```python
from build123d import *

# Parameters (mm, degrees)
SKETCH1_W           = 7.62
SKETCH1_H           = 7.62
BOSS_EXTRUDE1_DEPTH = 8.255
SKETCH3_R           = 1.5875
BOSS_EXTRUDE2_DEPTH = 6.35
SKETCH4_R           = 1.5875
BOSS_EXTRUDE3_DEPTH = 6.35


with BuildPart() as part:
    # Sketch1 → Boss-Extrude1 (new, symmetric)
    with BuildSketch(Plane.XY):
        Rectangle(SKETCH1_W, SKETCH1_H)
    extrude(amount=BOSS_EXTRUDE1_DEPTH, both=True)

    # Sketch2 → Cut-Revolve2 (revolve, cut)
    with BuildSketch(Plane(origin=(0, 0, 0), x_dir=(-1, 0, 0), z_dir=(0, -1, 0)), mode=Mode.PRIVATE) as cut_revolve2_sk:
        Polygon((-3.683, 8.255), (-12.573, 8.255), (-12.573, -8.255), (-3.683, -8.255), (-11.303, -3.855590949), (-11.303, 3.855590949), align=None)
    revolve(cut_revolve2_sk.sketch.rotate(Axis((0, 0, -8.255), (0, 0, 1)), 180), axis=Axis((0, 0, -8.255), (0, 0, 1)), mode=Mode.SUBTRACT)

    # Sketch3 → Boss-Extrude2 (add, symmetric)
    with BuildSketch(Plane.XZ):
        with Locations(Location((0, 0, 0), (0, 0, 90))):
            Circle(SKETCH3_R)
    extrude(amount=BOSS_EXTRUDE2_DEPTH, both=True)

    # Sketch4 → Boss-Extrude3 (add, symmetric)
    with BuildSketch(Plane.ZY):
        with Locations(Location((0, 0, 0), (0, 0, 180))):
            Circle(SKETCH4_R)
    extrude(amount=BOSS_EXTRUDE3_DEPTH, both=True)


solid = part.part
```
Can you work these out from the model? Positions are in its coordinate system, mm. A direction names the side the tool comes from. Coordinates: 2 decimals unless noted, no trailing zeros. Loops run counter-clockwise (first coordinate to the right, second up) from the corner with the lowest first, then second, coordinate; pieces in that order, holes last.
1) I need wall thicknesses on probe 1 along Y at (x, z) = (2.75, -0.25); probe 2 along X at (y, z) = (4.25, 1.25). Which ranges of each line are inside material? Lowest first, please.
2) Which directions (+Z, -Z, +X, -X, +Y, -Y) give clear straight access to the entire face, cutting with the end or side of a thin tool? Please do faces 1 (the cylindrical face through (5.06, 1.41, -0.73)), 2 (the flat face through (0, 6.35, 0)), 3 (the cylindrical face through (-5.1, 1.41, -0.73)), 4 (the cylindrical face through (0.966, -5.098, -1.26)), 5 (the cylindrical face through (0.966, 5.062, -1.26)).
3) Imagine slicing it at D-D on x = -5. List the corners of the cut face in (y, z) for me (1 decimal), plus the area to 3 significant figures.
4) Imagine slicing it at C-C on z = 0. List the corners of the cut face in (x, y) for me, plus the area to 3 significant figures.
5) For pin 1 (1 mm diameter, centred on x = 4.5, y = 0, fed in from -Z); pin 2 (4 mm diameter, centred on x = 4.5, y = -4, fed in from +Z); pin 3 (1.5 mm diameter, centred on y = 2, z = 2.5, fed in from -X), each with a flat end and sliding along its axis, tell me the tip position at first contact or that it passes through.
Completed:
1. probe 1: y = -3.81 to 3.81
1. probe 2: x = -0.98 to 0.98
2. face 1: +X
2. face 2: +Z, -Z, +X, -X, +Y
2. face 3: -X
2. face 4: -Y
2. face 5: +Y
3. outline: circle Ø3.2 at (0, 0)
3. area: 7.92 mm2
4. outline: (-6.35, -1.59) - (-3.81, -1.59) - (-3.81, -3.81) - (-1.59, -3.81) - (-1.59, -6.35) - (1.59, -6.35) - (1.59, -3.81) - (3.81, -3.81) - (3.81, -1.59) - (6.35, -1.59) - (6.35, 1.59) - (3.81, 1.59) - (3.81, 3.81) - (1.59, 3.81) - (1.59, 6.35) - (-1.59, 6.35) - (-1.59, 3.81) - (-3.81, 3.81) - (-3.81, 1.59) - (-6.35, 1.59) - close
4. area: 90.3 mm2
5. pin 1: stops at z = -1.59
5. pin 2: stops at z = 8.06
5. pin 3: stops at x = -3.81
